Here's how the part is built. I have some questions about the finished solid (model axes, mm). Face numbers are marked on the shaded views. A direction names the side the tool comes from. Coordinates: 2 decimals unless noted, no trailing zeros. Order: outer loops, then holes, each group sorted by start corner. A loop starts at its lowest first (then second) coordinate and runs counter-clockwise, first axis right, second up. Notation, with made-up numbers: (8.25, 54) - (54.25, 54) arc R6 cw to (54.25, 58) - close; hole circle Ø5 at (29.5, 38.5). An arc over 180 degrees is marked (long way). Answer as CSV lines item,"result". Start each with the question number.
Q1. For the marked faces 5 and 6, which set-ups out of +Z, -Z, +X, -X, +Y, -Y let a thin tool reach every point of the face, with its end or its side?
Q2. Suppose I cut it at A-A (x = 122). Please give me the cut outline in (y, z), then the cut area to 4 significant figures.
Q3. For pin 1 Ø5 at (y, z) = (83, 5.5) entering from +X; pin 2 Ø0.8 at (x, z) = (38, 30) entering from -Y; pin 3 Ø0.8 at (x, z) = (51, 30) entering from +Y; pin 4 Ø1.6 at (x, z) = (31, 29.5) entering from -Y, each with a flat end and sliding along its axis, tell me the tip position at first contact or that it passes through.
Q4. Suppose I cut it at C-C (z = -7). Please give me the cut outline in (x, y).
Q5. I need wall thicknesses on line 1 (Y direction, x = 17, z = -2.5); line 2 (X direction, y = 77, z = -1); line 3 (X direction, y = 10.5, z = -6.5). Which ranges of each line are inside material? Lowest first, please.
Q6. Suppose I cut it at B-B (y = -74.5). Please give me the cut outline in (x, z).
Q7. Thinking about a two-plate mould opening in Z: for the marked faces 1, 2, 3 and 4, which applies, released by +Z, released by -Z, zero draft, split by the parting line, or undercut?
Q8. Suppose I cut it at D-D (z = 18). Please give me the cut outline in (x, y).
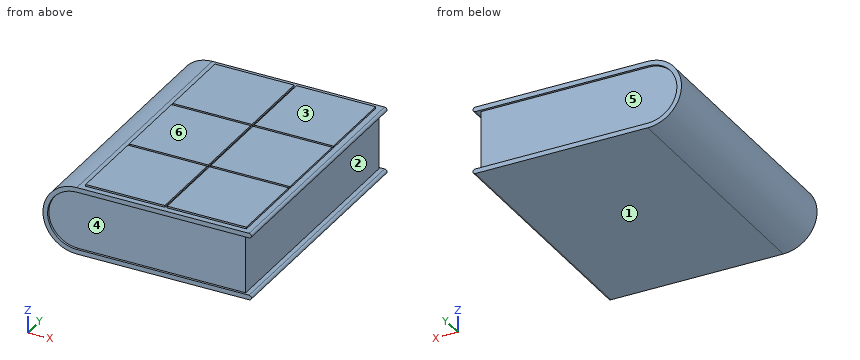
from build123d import *

# Parameters (mm, degrees)
F1_DEPTH = 109
F3_DEPTH = 107
F4_W     = 68
F4_H     = 68
F5_DEPTH = 1.5


# Not quite as in the source:
# - ends of sketch curves that miss each other by under 0.0002 mm in the source are joined


with BuildPart() as f1:
    # F0 (on Front) → F1 (new body, symmetric)
    with BuildSketch(Plane.XZ):
        with BuildLine():
            ThreePointArc((0, -25), (-25, 0), (0, 25))
            Line((0, 25), (148, 25))
            ThreePointArc((148, 25), (150, 26.9999995828), (148, 28.9999995828))
            Line((148, 28.9999995828), (0, 28.9999991655))
            ThreePointArc((0, 28.9999991655), (-28.9999991655, 0), (0, -28.9999991655))
            Line((0, -28.9999991655), (148, -28.9999991655))
            ThreePointArc((148, -28.9999991655), (150, -26.9999995828), (148, -24.9999995828))
            Line((148, -24.9999995828), (0, -25))
        make_face()
    extrude(amount=F1_DEPTH, both=True)

    # F2 (on Front) → F3 (join, symmetric)
    with BuildSketch(Plane.XZ):
        with BuildLine():
            Line((144, 25), (0, 25))
            ThreePointArc((0, 25), (-25, 0), (0, -25))
            Line((0, -25), (144, -25))
            Line((144, -25), (144, 25))
        make_face()
    extrude(amount=F3_DEPTH, both=True)

    # F4 (on face) → F5 (join)
    with BuildSketch(Plane.XY.offset(28.9999991655)):
        with Locations((39, 70)):
            Rectangle(F4_W, F4_H)
        with Locations((39, 0)):
            Rectangle(F4_W, F4_H)
        with Locations((39, -70)):
            Rectangle(F4_W, F4_H)
        with Locations((109, 70)):
            Rectangle(F4_W, F4_H)
        with Locations((109, 0)):
            Rectangle(F4_W, F4_H)
        with Locations((109, -70)):
            Rectangle(F4_W, F4_H)
    extrude(amount=F5_DEPTH)


solid = f1.part
Here are the results:
1,face 5,"+X, +Y"
1,face 6,"+Z, +X, -X, +Y, -Y"
2,outline,"(-109, -29) - (109, -29) - (109, -25) - (107, -25) - (107, 25) - (109, 25) - (109, 29) - (104, 29) - (104, 30.5) - (36, 30.5) - (36, 29) - (34, 29) - (34, 30.5) - (-34, 30.5) - (-34, 29) - (-36, 29) - (-36, 30.5) - (-104, 30.5) - (-104, 29) - (-109, 29) - (-109, 25) - (-107, 25) - (-107, -25) - (-109, -25) - close"
2,area,"12,750 mm²"
3,pin 1,"stops at x = 144"
3,pin 2,"stops at y = -104"
3,pin 3,"stops at y = 104"
3,pin 4,"stops at y = -109"
4,outline,"(-28.14, -109) - (-24, -109) - (-24, -107) - (144, -107) - (144, 107) - (-24, 107) - (-24, 109) - (-28.14, 109) - close"
5,line 1,"y = -107 to 107"
5,line 2,"x = -28.98 to 144"
5,line 3,"x = -28.26 to 144"
6,outline,"(0, -29) - (148, -29) arc R2 ccw to (148, -25) - (144, -25) - (144, 25) - (148, 25) arc R2 ccw to (148, 29) - (143, 29) - (143, 30.5) - (75, 30.5) - (75, 29) - (73, 29) - (73, 30.5) - (5, 30.5) - (5, 29) - (0, 29) arc R29 ccw to start"
7,face 1,"released by -Z"
7,face 2,"undercut"
7,face 3,"released by +Z"
7,face 4,"undercut"
8,outline,"(-22.74, -109) - (-17.35, -109) - (-17.35, -107) - (144, -107) - (144, 107) - (-17.35, 107) - (-17.35, 109) - (-22.74, 109) - close"
